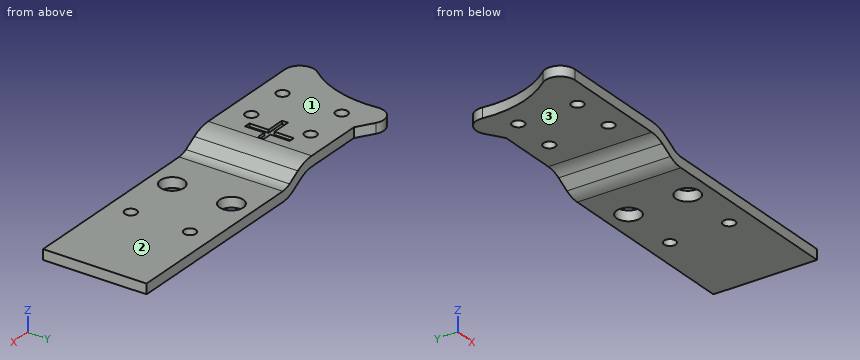
from build123d import *

# Parameters (mm, degrees)
BOSS_EXTRUDE1_DEPTH = 3.4
SKETCH3_R           = 5
CUT_EXTRUDE1_DEPTH  = 6
CUT_EXTRUDE2_DEPTH  = 10
SKETCH6_R           = 35
CUT_EXTRUDE3_DEPTH  = 10
CUT_EXTRUDE4_DEPTH  = 1
CUT_EXTRUDE5_REACH  = 87.508
SKETCH8_W           = 12
SKETCH8_H           = 35
BOSS_EXTRUDE2_DEPTH = 35
SKETCH10_R          = 4
CUT_EXTRUDE6_DEPTH  = 10
CUT_EXTRUDE7_REACH  = 153.093
SKETCH11_R          = 2
CUT_EXTRUDE8_REACH  = 153.243
SKETCH12_R          = 2
FILLET1_R           = 5


with BuildPart() as part:
    # Sketch1 → Boss-Extrude1 (new body)
    with BuildSketch(Plane.XY):
        with BuildLine():
            Line((0, -30), (80, -30))
            Line((80, -30), (80, 5))
            Line((80, 5), (48, 5))
            Line((48, 5), (16.114075804, 25.304872277))
            ThreePointArc((16.114075804, 25.304872277), (-28.802310396, 8.392074585), (0, -30))
        make_face()
    extrude(amount=BOSS_EXTRUDE1_DEPTH)

    # Sketch3 → Cut-Extrude1 (cut)
    with BuildSketch(Plane.XY.offset(3.4)):
        Circle(SKETCH3_R)
    extrude(amount=-CUT_EXTRUDE1_DEPTH, mode=Mode.SUBTRACT)

    # Sketch5 → Cut-Extrude2 (cut)
    with BuildSketch(Plane.XY.offset(3.4)):
        with BuildLine():
            ThreePointArc((0, 10), (-8.660254038, 5), (-8.660254038, -5))
            ThreePointArc((-8.660254038, -5), (-10.124355653, -10.464101615), (-15.588457268, -9))
            ThreePointArc((-15.588457268, -9), (-15.588457268, 9), (0, 18))
            ThreePointArc((0, 18), (4, 14), (0, 10))
        make_face()
    extrude(amount=-CUT_EXTRUDE2_DEPTH, mode=Mode.SUBTRACT)

    # Sketch6 → Cut-Extrude3 (cut)
    with BuildSketch(Plane(origin=(0, 0, 0), x_dir=(-1, 0, 0), z_dir=(0, 0, -1))):
        Circle(SKETCH6_R)
    extrude(amount=-CUT_EXTRUDE3_DEPTH, mode=Mode.SUBTRACT)

    # Sketch7 → Cut-Extrude4 (cut)
    with BuildSketch(Plane.XY.offset(3.4)):
        Polygon((62.77538264, -13.5), (62.77538264, -20), (64.77538264, -20), (64.77538264, -13.5), (71.27538264, -13.5), (71.27538264, -11.5), (64.77538264, -11.5), (64.77538264, -5), (62.77538264, -5), (62.77538264, -11.5), (56.27538264, -11.5), (56.27538264, -13.5), align=None)
    extrude(amount=-CUT_EXTRUDE4_DEPTH, mode=Mode.SUBTRACT)

    # Sketch8 → Cut-Extrude5 (cut, up to next)
    with BuildSketch(Plane(origin=(0, 0, 0), x_dir=(-1, 0, 0), z_dir=(0, 0, -1)), mode=Mode.PRIVATE) as cut_extrude5_sk1:
        with Locations((-74, -12.5)):
            Rectangle(SKETCH8_W, SKETCH8_H)
    cut_extrude5_tool1 = extrude(cut_extrude5_sk1.sketch, amount=-CUT_EXTRUDE5_REACH, mode=Mode.PRIVATE) & part.part
    add(cut_extrude5_tool1.solids().sort_by_distance((74, -12.5, 0))[0], mode=Mode.SUBTRACT)

    # Sketch9 → Boss-Extrude2 (add)
    with BuildSketch(Plane(origin=(0, 5, 0), x_dir=(1, 0, 0), z_dir=(0, 1, 0))):
        with BuildLine():
            Line((68, 0), (68.320508076, 0))
            ThreePointArc((68.320508076, 0), (70.908698527, 0.340741737), (73.320508076, 1.339745962))
            Line((73.320508076, 1.339745962), (77.339745962, 3.660254038))
            ThreePointArc((77.339745962, 3.660254038), (79.751555511, 4.659258263), (82.339745962, 5))
            Line((82.339745962, 5), (83, 5))
            Line((83, 5), (148, 5))
            Line((148, 5), (148, 1.6))
            Line((148, 1.6), (83, 1.6))
            Line((83, 1.6), (82.339745962, 1.6))
            ThreePointArc((82.339745962, 1.6), (80.631540264, 1.375110454), (79.039745962, 0.715767665))
            Line((79.039745962, 0.715767665), (75.020508076, -1.604740411))
            ThreePointArc((75.020508076, -1.604740411), (71.78868328, -2.943406072), (68.320508076, -3.4))
            Line((68.320508076, -3.4), (68, -3.4))
            Line((68, -3.4), (68, 0))
        make_face()
    extrude(amount=-BOSS_EXTRUDE2_DEPTH)

    # Sketch10 → Cut-Extrude6 (cut)
    with BuildSketch(Plane(origin=(0, 0, -5), x_dir=(-1, 0, 0), z_dir=(0, 0, -1))):
        with Locations((-96.339745962, -2.5)):
            Circle(SKETCH10_R)
        with Locations(Location((-96.339745962, -22.5, 0), (0, 0, 180))):
            Circle(SKETCH10_R)
    extrude(amount=-CUT_EXTRUDE6_DEPTH, mode=Mode.SUBTRACT)

    # Sketch11 → Cut-Extrude7 (cut, up to next)
    with BuildSketch(Plane(origin=(0, 0, 0), x_dir=(-1, 0, 0), z_dir=(0, 0, -1)), mode=Mode.PRIVATE) as cut_extrude7_sk1:
        with Locations((-58.160254038, -22.5)):
            Circle(SKETCH11_R)
    cut_extrude7_tool1 = extrude(cut_extrude7_sk1.sketch, amount=-CUT_EXTRUDE7_REACH, mode=Mode.PRIVATE) & part.part
    # Sketch11 → Cut-Extrude7 (cut, up to next)
    with BuildSketch(Plane(origin=(0, 0, 0), x_dir=(-1, 0, 0), z_dir=(0, 0, -1)), mode=Mode.PRIVATE) as cut_extrude7_sk2:
        with Locations((-58.160254038, -2.5)):
            Circle(SKETCH11_R)
    cut_extrude7_tool2 = extrude(cut_extrude7_sk2.sketch, amount=-CUT_EXTRUDE7_REACH, mode=Mode.PRIVATE) & part.part
    # Sketch11 → Cut-Extrude7 (cut, up to next)
    with BuildSketch(Plane(origin=(0, 0, 0), x_dir=(-1, 0, 0), z_dir=(0, 0, -1)), mode=Mode.PRIVATE) as cut_extrude7_sk3:
        with Locations((-43.160254038, -22.5)):
            Circle(SKETCH11_R)
    cut_extrude7_tool3 = extrude(cut_extrude7_sk3.sketch, amount=-CUT_EXTRUDE7_REACH, mode=Mode.PRIVATE) & part.part
    # Sketch11 → Cut-Extrude7 (cut, up to next)
    with BuildSketch(Plane(origin=(0, 0, 0), x_dir=(-1, 0, 0), z_dir=(0, 0, -1)), mode=Mode.PRIVATE) as cut_extrude7_sk4:
        with Locations((-43.160254038, -2.5)):
            Circle(SKETCH11_R)
    cut_extrude7_tool4 = extrude(cut_extrude7_sk4.sketch, amount=-CUT_EXTRUDE7_REACH, mode=Mode.PRIVATE) & part.part
    add(cut_extrude7_tool1.solids().sort_by_distance((58.160254, -22.5, 0))[0], mode=Mode.SUBTRACT)
    add(cut_extrude7_tool2.solids().sort_by_distance((58.160254, -2.5, 0))[0], mode=Mode.SUBTRACT)
    add(cut_extrude7_tool3.solids().sort_by_distance((43.160254, -22.5, 0))[0], mode=Mode.SUBTRACT)
    add(cut_extrude7_tool4.solids().sort_by_distance((43.160254, -2.5, 0))[0], mode=Mode.SUBTRACT)

    # Sketch12 → Cut-Extrude8 (cut, up to next)
    with BuildSketch(Plane(origin=(0, 0, -5), x_dir=(-1, 0, 0), z_dir=(0, 0, -1)), mode=Mode.PRIVATE) as cut_extrude8_sk1:
        with Locations((-116.339745962, -22.5)):
            Circle(SKETCH12_R)
    cut_extrude8_tool1 = extrude(cut_extrude8_sk1.sketch, amount=-CUT_EXTRUDE8_REACH, mode=Mode.PRIVATE) & part.part
    # Sketch12 → Cut-Extrude8 (cut, up to next)
    with BuildSketch(Plane(origin=(0, 0, -5), x_dir=(-1, 0, 0), z_dir=(0, 0, -1)), mode=Mode.PRIVATE) as cut_extrude8_sk2:
        with Locations((-116.339745962, -2.5)):
            Circle(SKETCH12_R)
    cut_extrude8_tool2 = extrude(cut_extrude8_sk2.sketch, amount=-CUT_EXTRUDE8_REACH, mode=Mode.PRIVATE) & part.part
    add(cut_extrude8_tool1.solids().sort_by_distance((116.339746, -22.5, -5))[0], mode=Mode.SUBTRACT)
    add(cut_extrude8_tool2.solids().sort_by_distance((116.339746, -2.5, -5))[0], mode=Mode.SUBTRACT)

    # Fillet1
    fillet1_edges = [part.edges().sort_by_distance(p)[0] for p in [
        (31.320411557, 15.621517849, 1.7),
        (18.027756377, -30, 1.7),
    ]]
    fillet(fillet1_edges, radius=FILLET1_R)


solid = part.part
The listing builds one solid part. Answer for the finished solid, in the listing's coordinates (mm). Face numbers are marked on the shaded views. A direction names the side the tool comes from. Round coordinates to 2 decimals unless told otherwise and drop trailing zeros. Loops run counter-clockwise (first coordinate to the right, second up) from the corner with the lowest first, then second, coordinate; pieces in that order, holes last. Notation, with made-up numbers: M -36.75,-30 L 7.25,-30 A16 ccw 7.25,-21 Z; hole C 33,-35 d11. An arc over 180 degrees is marked long. Return JSON: item names as keys, results as strings.
Q1. Find the intervals of material crossed by line 1 along Y through (x, z) = (58.5, 0.75); line 2 along Y through (x, z) = (94.5, -2); line 3 along Z through (x, y) = (137, -14), in increasing order. Write a range as from..to.
Results list:
{"line 1": "y = -30..-24.47, -20.53..-4.47, -0.53..5", "line 2": "y = -30..-26.05, -18.95..-6.05, 1.05..5", "line 3": "z = -5..-1.6"}
Q2. Find section D-D, the plane x = 110. Determine the outline of the cut face in (y, z), plus the area to 3 significant figures.
Results list:
{"outline": "M -30,-5 L 5,-5 L 5,-1.6 L -30,-1.6 Z", "area": "119 mm2"}
Q3. Find section A-A, the plane y = -2.5. Determine the outline of the cut face in (x, z).
Results list:
{"outline": "M 34.91,0 L 41.16,0 L 41.16,3.4 L 34.91,3.4 Z; M 45.16,0 L 56.16,0 L 56.16,3.4 L 45.16,3.4 Z; M 60.16,0 L 68.32,0 A10 cw 73.32,-1.34 L 77.34,-3.66 A10 ccw 82.34,-5 L 92.34,-5 L 92.34,-1.6 L 82.34,-1.6 A6.6 cw 79.04,-0.72 L 75.02,1.6 A13.4 ccw 68.32,3.4 L 60.16,3.4 Z; M 100.34,-5 L 114.34,-5 L 114.34,-1.6 L 100.34,-1.6 Z; M 118.34,-5 L 148,-5 L 148,-1.6 L 118.34,-1.6 Z"}
Q4. Find section B-B, the plane x = 59. Determine the outline of the cut face in (y, z), plus the area to 3 significant figures.
Results list:
{"outline": "M -30,0 L -24.32,0 L -24.32,3.4 L -30,3.4 Z; M -20.68,0 L -4.32,0 L -4.32,3.4 L -11.5,3.4 L -11.5,2.4 L -13.5,2.4 L -13.5,3.4 L -20.68,3.4 Z; M -0.68,0 L 5,0 L 5,3.4 L -0.68,3.4 Z", "area": "92.3 mm2"}
Q5. Each of these flat-tipped pins is pushed along its axis until it touches: pin 1 Ø1.1 at (y, z) = (-9, 3) entering from -X; pin 2 Ø3 at (x, z) = (135.5, -2) entering from +Y; pin 3 Ø2 at (y, z) = (0, 2) entering from +X. Where does it stop, or does it pass through?
Results list:
{"pin 1": "stops at x = 33.67", "pin 2": "stops at y = 5", "pin 3": "stops at x = 76.07"}
Q6. Find section C-C, the plane y = -16. Determine the outline of the cut face in (x, z), plus the area to 3 significant figures.
Results list:
{"outline": "M 31.13,0 L 68.32,0 A10 cw 73.32,-1.34 L 77.34,-3.66 A10 ccw 82.34,-5 L 148,-5 L 148,-1.6 L 82.34,-1.6 A6.6 cw 79.04,-0.72 L 75.02,1.6 A13.4 ccw 68.32,3.4 L 64.78,3.4 L 64.78,2.4 L 62.78,2.4 L 62.78,3.4 L 31.13,3.4 Z", "area": "399 mm2"}
Q7. Which of the six approach directions +Z, -Z, +X, -X, +Y, -Y give full straight-line access (tool end or side, diameter ignored) to the marked faces 1, 2 and 3?
Results list:
{"face 1": "+Z, +X, -X, +Y, -Y", "face 2": "+Z, +X, +Y, -Y", "face 3": "-Z, -X, +Y, -Y"}
